Input: dimensioned drawing with shaded views. Units: mm. Origin: part minimum x, y, z. A direction names the side the tool comes from. Round coordinates to 2 decimals unless told otherwise and drop trailing zeros. Loops run counter-clockwise (first coordinate to the right, second up) from the corner with the lowest first, then second, coordinate; pieces in that order, holes last. Notation, with made-up numbers: (89.5, 17.5) -> (145.5, 17.5) arc R13 ccw to (145.5, 42.5) -> close; hole circle Ø10 at (18.25, -18). An arc over 180 degrees is marked (long way). Answer as a JSON object with one key per item and string values.
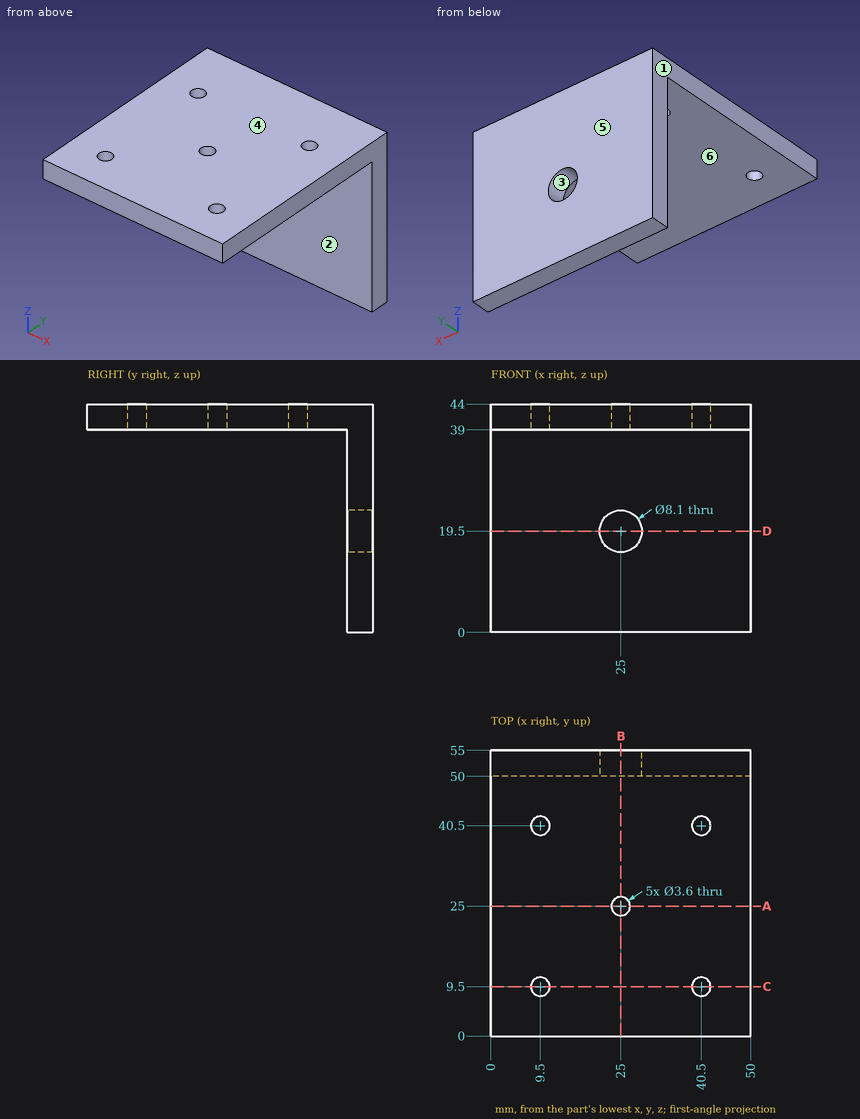
1) Contact query for flat-ended pins moving along their axis: P1, Ø3, axis at y = 16, z = 39, coming from the -X side; P2, Ø10.5, axis at x = 25, z = 19.5, coming from the -Y side; P3, Ø15, axis at x = 13, y = 21, coming from the -Z side. Output: stop coordinate, or through.
Output:
{"P1": "stops at x = 0", "P2": "stops at y = 50", "P3": "stops at z = 39"}
2) Section C-C, the plane y = 9.5. Output: boundary loops of the cut face in (x, z), plus the area to 3 significant figures.
Output:
{"outline": "(0, 39) -> (7.7, 39) -> (7.7, 44) -> (0, 44) -> close; (11.3, 39) -> (38.7, 39) -> (38.7, 44) -> (11.3, 44) -> close; (42.3, 39) -> (50, 39) -> (50, 44) -> (42.3, 44) -> close", "area": "214 mm^2"}
3) Draft query along Z for the marked faces 3, 4, 5 and 6. Return one class per face: +Z half, -Z half, draft (parallel to the pull), parting line (faces both ways), or undercut.
Output:
{"face 3": "undercut", "face 4": "+Z half", "face 5": "draft", "face 6": "-Z half"}
4) Section D-D, the plane z = 19.5. Output: boundary loops of the cut face in (x, y).
Output:
{"outline": "(0, 50) -> (20.95, 50) -> (20.95, 55) -> (0, 55) -> close; (29.05, 50) -> (50, 50) -> (50, 55) -> (29.05, 55) -> close"}
5) Ray query, probe 1 along Y at (x, z) = (40.5, 42.3); probe 2 along X at (y, z) = (40, 42); probe 3 along Z at (x, y) = (28.5, 30). Return the intervals inside material, ascending.
Output:
{"probe 1": "y = 0 to 7.7, 11.3 to 38.7, 42.3 to 55", "probe 2": "x = 0 to 7.77, 11.23 to 38.77, 42.23 to 50", "probe 3": "z = 39 to 44"}
6) Section A-A, the plane y = 25. Output: boundary loops of the cut face in (x, z).
Output:
{"outline": "(0, 39) -> (23.2, 39) -> (23.2, 44) -> (0, 44) -> close; (26.8, 39) -> (50, 39) -> (50, 44) -> (26.8, 44) -> close"}
7) Section B-B, the plane x = 25. Output: boundary loops of the cut face in (y, z), plus the area to 4 significant figures.
Output:
{"outline": "(0, 39) -> (23.2, 39) -> (23.2, 44) -> (0, 44) -> close; (26.8, 39) -> (50, 39) -> (50, 23.55) -> (55, 23.55) -> (55, 44) -> (26.8, 44) -> close; (50, 0) -> (55, 0) -> (55, 15.45) -> (50, 15.45) -> close", "area": "411.5 mm^2"}
8) Reachability of the marked faces 1 and 2 from +Z, -Z, +X, -X, +Y, -Y: full face, straight path, thin tool, end or side. Return the list, or none.
Output:
{"face 1": "+Z, -Z, -X, +Y, -Y", "face 2": "-Z, +X, -X, -Y"}
